Design review of the part built by this model. Coordinates are the model's own, in mm. Coordinates: 2 decimals unless noted, no trailing zeros. Write each loop counter-clockwise with the first axis right and the second up, starting at its lowest first coordinate (ties: lowest second). Pieces come first, ordered by that corner, then holes. Notation, with made-up numbers: (30.5, -1.5) -> (61.5, -1.5) arc R17 cw to (61.5, 15.5) -> close; hole circle Ø4 at (18, -5.5). An arc over 180 degrees is marked (long way). Answer in a Markdown table with one row per item. Add a question column.
Item 1: Take a section at B-B, the plane x = 87.5. Write out the cut boundary in (y, z).
Item 2: To check wall thickness, follow line 1 (X direction, y = 19, z = 0.75); line 2 (Y direction, x = 33.4, z = 2); line 3 (Y direction, x = 1, z = 2.55). State the ranges of each line that lie inside material, in increasing order.
Item 3: Take a section at A-A, the plane z = 1.9. Give the number of separate pieces and of enclosed holes in the cut face, and give its area (3 significant figures).
Item 4: Clearance check with flat-ended pins moving along their axes: P1, Ø1.9, axis at y = -15, z = 1, coming from the -X side; P2, Ø1.1, axis at y = -19, z = 2, coming from the +X side; P3, Ø1.1, axis at x = 227, z = 2, coming from the -Y side. State where each tip first meets the part, or that it passes through.
from build123d import *

# Parameters (mm, degrees)
SKETCH1_R           = 1.75
SKETCH1_R_2         = 2.25
SKETCH1_R_3         = 1.5
BOSS_EXTRUDE1_DEPTH = 3.8


with BuildPart() as part:
    # Sketch1 → Boss-Extrude1 (new body)
    with BuildSketch(Plane.XY):
        with BuildLine():
            Line((299, -10.001863855), (156.039811852, -10.001863855))
            ThreePointArc((156.039811852, -10.001863855), (155.33270507, -10.294757074), (155.039811852, -11.001863855))
            Line((155.039811852, -11.001863855), (155.039811852, -22.458474266))
            ThreePointArc((155.039811852, -22.458474266), (153.868238976, -25.286901391), (151.039811852, -26.458474266))
            Line((151.039811852, -26.458474266), (110.724043242, -26.458474266))
            ThreePointArc((110.724043242, -26.458474266), (107.895616117, -25.286901391), (106.724043242, -22.458474266))
            Line((106.724043242, -22.458474266), (106.724043242, -11.001863855))
            ThreePointArc((106.724043242, -11.001863855), (106.431150023, -10.294757074), (105.724043242, -10.001863855))
            Line((105.724043242, -10.001863855), (-9, -10.001863855))
            ThreePointArc((-9, -10.001863855), (-9.707106781, -9.708970637), (-10, -9.001863855))
            Line((-10, -9.001863855), (-10, 60))
            ThreePointArc((-10, 60), (-9.707106781, 60.707106781), (-9, 61))
            Line((-9, 61), (299, 61))
            ThreePointArc((299, 61), (299.707106781, 60.707106781), (300, 60))
            Line((300, 60), (300, -9.001863855))
            ThreePointArc((300, -9.001863855), (299.707106781, -9.708970637), (299, -10.001863855))
        make_face()
        with Locations(Location((289, 22.001504258, 0), (0, 0, 180))):
            Circle(SKETCH1_R, mode=Mode.SUBTRACT)
        with Locations(Location((289, 47.001504258, 0), (0, 0, 180))):
            Circle(SKETCH1_R, mode=Mode.SUBTRACT)
        with Locations(Location((148.082820817, -11.316051766, 0), (0, 0, 180))):
            Circle(SKETCH1_R_2, mode=Mode.SUBTRACT)
        with Locations(Location((148.082820817, 13.683948234, 0), (0, 0, 180))):
            Circle(SKETCH1_R_2, mode=Mode.SUBTRACT)
        with Locations(Location((114.224914373, 13.683948234, 0), (0, 0, 180))):
            Circle(SKETCH1_R_2, mode=Mode.SUBTRACT)
        with Locations(Location((114.224914373, -11.316051766, 0), (0, 0, 180))):
            Circle(SKETCH1_R_2, mode=Mode.SUBTRACT)
        with Locations(Location((256.6, 19.147207957, 0), (0, 0, 180))):
            Circle(SKETCH1_R_3, mode=Mode.SUBTRACT)
        with Locations(Location((270.5, 19.147207957, 0), (0, 0, 180))):
            Circle(SKETCH1_R_3, mode=Mode.SUBTRACT)
        with Locations(Location((270.5, 34.947207957, 0), (0, 0, 180))):
            Circle(SKETCH1_R_3, mode=Mode.SUBTRACT)
        with Locations(Location((256.6, 34.947207957, 0), (0, 0, 180))):
            Circle(SKETCH1_R_3, mode=Mode.SUBTRACT)
        with Locations(Location((33.4, 34.947207957, 0), (0, 0, 180))):
            Circle(SKETCH1_R_3, mode=Mode.SUBTRACT)
        with Locations(Location((19.5, 34.947207957, 0), (0, 0, 180))):
            Circle(SKETCH1_R_3, mode=Mode.SUBTRACT)
        with Locations(Location((19.5, 19.147207957, 0), (0, 0, 180))):
            Circle(SKETCH1_R_3, mode=Mode.SUBTRACT)
        with Locations(Location((33.4, 19.147207957, 0), (0, 0, 180))):
            Circle(SKETCH1_R_3, mode=Mode.SUBTRACT)
        with Locations(Location((1, 47.001504258, 0), (0, 0, 180))):
            Circle(SKETCH1_R, mode=Mode.SUBTRACT)
        with Locations(Location((1, 22.001504258, 0), (0, 0, 180))):
            Circle(SKETCH1_R, mode=Mode.SUBTRACT)
    extrude(amount=BOSS_EXTRUDE1_DEPTH)


solid = part.part
Answers:
| question | item | result |
|---|---|---|
| 1 | outline | (-10, 0) -> (61, 0) -> (61, 3.8) -> (-10, 3.8) -> close |
| 2 | line 1 | x = -10 to 18.01, 20.99 to 31.91, 34.89 to 255.11, 258.09 to 269.01, 271.99 to 300 |
| 2 | line 2 | y = -10 to 17.65, 20.65 to 33.45, 36.45 to 61 |
| 2 | line 3 | y = -10 to 20.25, 23.75 to 45.25, 48.75 to 61 |
| 3 | separate pieces | 1 |
| 3 | enclosed holes | 16 |
| 3 | area | 22,600 mm^2 |
| 4 | P1 | stops at x = 106.72 |
| 4 | P2 | stops at x = 155.04 |
| 4 | P3 | stops at y = -10 |
